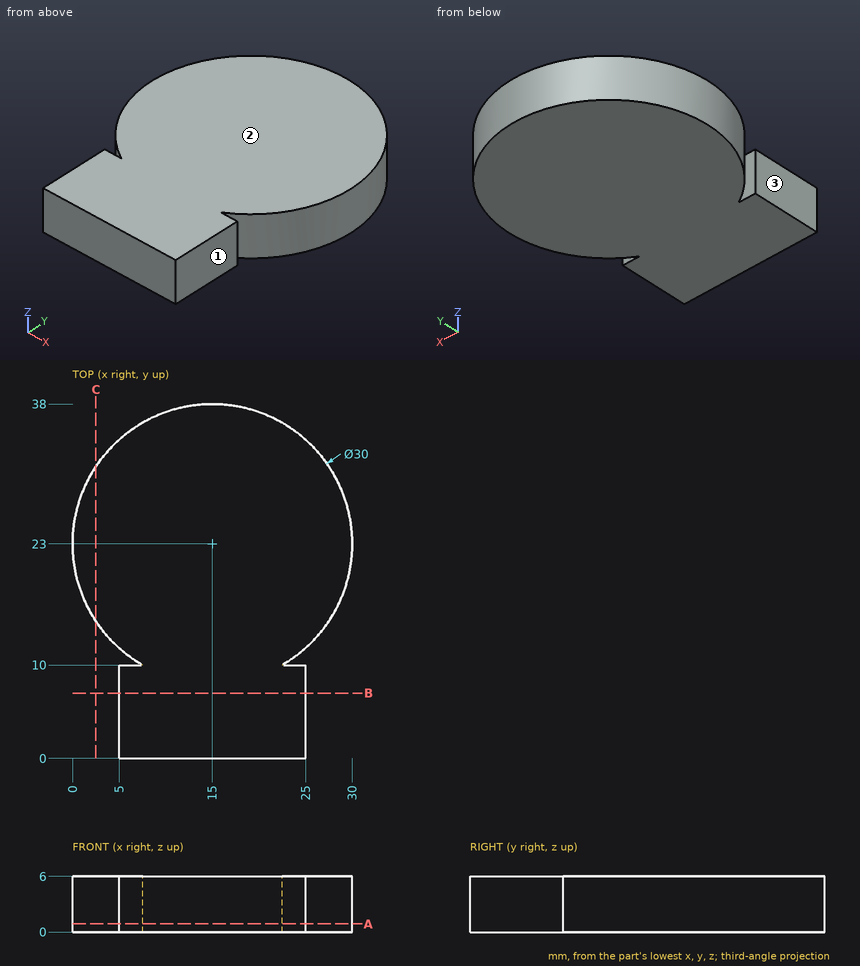
Design review of the part shown in the three views and the two pictorial views. Dimensions are in mm from the part's minimum x, y and z. A direction names the side the tool comes from. Give positions to 0.01 mm unless a question says otherwise; leave off trailing zeros. Loops run counter-clockwise (first coordinate to the right, second up) from the corner with the lowest first, then second, coordinate; pieces in that order, holes last. Notation, with made-up numbers: (57.5, 19) -> (95.5, 19) arc R27 ccw to (95.5, 46) -> close; hole circle Ø11 at (33.5, 32.5). An arc over 180 degrees is marked (long way). One line per item, written item: value.
Q1. We need section B-B on y = 7. Give the boundary of the cut face in (x, z), and give its area (3 significant figures).
Numbers:
outline: (5, 0) -> (25, 0) -> (25, 6) -> (5, 6) -> close
area: 120 mm^2
Q2. We need section C-C on x = 2.5. Give the boundary of the cut face in (y, z).
Numbers:
outline: (14.71, 0) -> (31.29, 0) -> (31.29, 6) -> (14.71, 6) -> close
Q3. We need section A-A on z = 0.9. Give the boundary of the cut face in (x, y), and give its area (3 significant figures).
Numbers:
outline: (5, 0) -> (25, 0) -> (25, 10) -> (22.48, 10) arc R15 ccw (long way) to (7.52, 10) -> (5, 10) -> close
area: 887 mm^2
Q4. For L1, parallel to X at y = 22.5, z = 4.3; L2, parallel to Y at x = 22.75, z = 5.55; L3, parallel to X at y = 14, z = 3.1, list the stretches that pass through material, from the lowest coordinate up.
Numbers:
L1: x = 0.01 to 29.99
L2: y = 0 to 10, 10.16 to 35.84
L3: x = 3 to 27
Q5. Machinability: for the marked faces 1, 2 and 3, which of the approach directions +Z, -Z, +X, -X, +Y, -Y give a long, thin tool a straight path to every point of the face, cutting with its end or side? Answer none if there is none.
Numbers:
face 1: +Z, -Z, +X, -Y
face 2: +Z, +X, -X, +Y, -Y
face 3: +Z, -Z, -X, -Y
Q6. For pin 1 Ø1 at (x, z) = (17.5, 3) entering from -Y; pin 2 Ø3 at (x, z) = (25.5, 3) entering from +Y; pin 3 Ø1.3 at (x, z) = (6.5, 3.5) entering from +Y; pin 4 Ø3 at (y, z) = (20, 2) entering from +X, all flat-tipped, find the tip position at first contact; note any pin that passes through.
Numbers:
pin 1: stops at y = 0
pin 2: stops at y = 35
pin 3: stops at y = 35.78
pin 4: stops at x = 29.92
